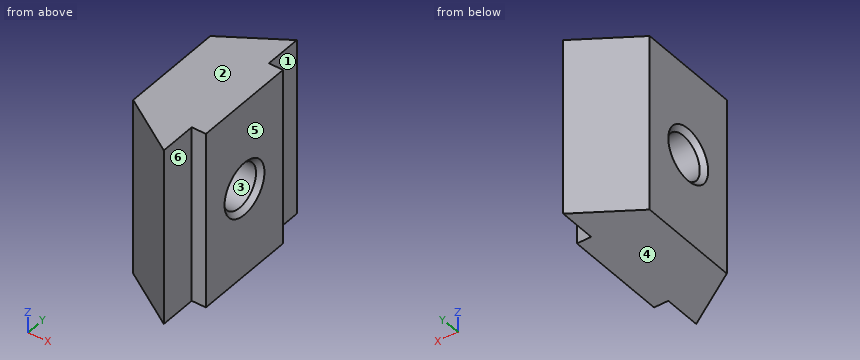
Autodesk Inventor part; units mm, degrees
ref_plane "nut_XY" through (0, 0, 0) normal (1, 0, 0) x (0, 0, -1)
ref_plane "nut_YZ" through (0, 0, 0) normal (0, 0, -1) x (0, 1, 0)
ref_plane "nut_ZX" through (0, 0, 0) normal (0, 1, 0) x (1, 0, 0)
sketch "Sketch_4" plane through (0, 0, 0) normal (0, 0, 1) x (1, 0, 0)
  line L0 (-4.1, 2.9) -> (-4.1, -2.9)
  line L1 (-4.1, -2.9) -> (-0.8, -5)
  line L2 (-0.8, -5) -> (-0.8, -2.9)
  line L3 (-0.8, -2.9) -> (0, -2.9)
  line L4 (0, -2.9) -> (0, 2.9)
  line L5 (0, 2.9) -> (-0.8, 2.9)
  line L6 (-0.8, 2.9) -> (-0.8, 5)
  line L7 (-0.8, 5) -> (-4.1, 2.9)
extrude "Extrusion1" add sketch "Sketch_4" along normal mid plane 10
sketch "Sketch_5" plane through (0, 0, 0) normal (0, 0, 1) x (1, 0, 0)
  line L0 (0, 0) -> (-4.1, 0)
  line L1 (-4.1, 0) -> (-4.1, 1.5)
  line L2 (-4.1, 1.5) -> (-3.8295, 1.2295)
  line L3 (-3.8295, 1.2295) -> (-0.2705, 1.2295)
  line L4 (-0.2705, 1.2295) -> (0, 1.5)
  line L5 (0, 1.5) -> (0, 0)
  line L6 (0, 0) -> (-4.1, 0)
revolve "Revolution1" cut sketch "Sketch_5" angle 360 about axis through (0, 0, 0) along (1, 0, 0)
thread "Thread1"
ref_plane "nut_XY" through (0, 0, 0) normal (1, 0, 0) x (0, 0, -1)
ref_plane "nut_YZ" through (0, 0, 0) normal (0, 0, -1) x (0, 1, 0)
ref_plane "nut_ZX" through (0, 0, 0) normal (0, 1, 0) x (1, 0, 0)
ref_plane "to_bolt_XY" through (-4.1, 0, 0) normal (1, 0, 0) x (0, 0, -1)
ref_plane "to_bolt_YZ" through (-4.1, 0, 0) normal (0, 0, -1) x (0, 1, 0)
ref_plane "to_bolt_ZX" through (-4.1, 0, 0) normal (0, 1, 0) x (1, 0, 0)
ref_plane "to_frames_XY" through (-0.8, 0, 0) normal (1, 0, 0) x (0, 0, -1)
ref_plane "to_frames_YZ" through (-0.8, 0, 0) normal (0, 0, -1) x (0, 1, 0)
ref_plane "to_frames_ZX" through (-0.8, 0, 0) normal (0, 1, 0) x (1, 0, 0)
properties part number "HNTT5-3_1"
Input: part model. Units: mm. Frame: model coordinates. Face numbers are marked on the shaded views. A direction names the side the tool comes from. Coordinates: 2 decimals unless noted, no trailing zeros. Order: outer loops, then holes, each group sorted by start corner. A loop starts at its lowest first (then second) coordinate and runs counter-clockwise, first axis right, second up.
1. Cut plane A-A, the plane y = 0. Return loops of the section in (x, z).
Checked values:
outline: (-4.1, -5) - (0, -5) - (0, -1.5) - (-0.27, -1.23) - (-3.83, -1.23) - (-4.1, -1.5) - close; (-4.1, 1.5) - (-3.83, 1.23) - (-0.27, 1.23) - (0, 1.5) - (0, 5) - (-4.1, 5) - close
2. Cut plane B-B, the plane z = 0. Return loops of the section in (x, y).
Checked values:
outline: (-4.1, -2.9) - (-0.8, -5) - (-0.8, -2.9) - (0, -2.9) - (0, -1.5) - (-0.27, -1.23) - (-3.83, -1.23) - (-4.1, -1.5) - close; (-4.1, 1.5) - (-3.83, 1.23) - (-0.27, 1.23) - (0, 1.5) - (0, 2.9) - (-0.8, 2.9) - (-0.8, 5) - (-4.1, 2.9) - close
3. Ray query, line 1 along Z through (x, y) = (-1.25, 0); line 2 along Y through (x, z) = (-0.5, -2.5); line 3 along Z through (x, y) = (-1.55, -0.5). Return the intervals inside material, ascending.
Checked values:
line 1: z = -5 to -1.23, 1.23 to 5
line 2: y = -2.9 to 2.9
line 3: z = -5 to -1.12, 1.12 to 5
4. Cut plane C-C, the plane x = -3.35. Return loops of the section in (y, z), plus the area to 3 significant figures.
Checked values:
outline: (-3.38, -5) - (3.38, -5) - (3.38, 5) - (-3.38, 5) - close; hole circle Ø2.46 at (0, 0)
area: 62.8 mm2
5. Access query for the marked faces 5 and 6. Directions: +Z, -Z, +X, -X, +Y, -Y. A direction counts if a zero-diameter tool reaches every point of the face in a straight line with its end or side. Return the directions, or none.
Checked values:
face 5: +Z, -Z, +X, +Y, -Y
face 6: +Z, -Z, +X, -Y
6. Contact query for flat-ended pins moving along their axis: P1, Ø2, axis at x = -3.5, z = 3, coming from the +Y side; P2, Ø0.9, axis at x = -0.5, z = 1.5, coming from the -Y side. Output: stop coordinate, or through.
Checked values:
P1: stops at y = 3.92
P2: stops at y = -5
7. Draft query along Z for the marked faces 1, 2, 3 and 4. Return one class per face: +Z half, -Z half, draft (parallel to the pull), parting line (faces both ways), or undercut.
Checked values:
face 1: draft
face 2: +Z half
face 3: undercut
face 4: -Z half
8. Cut plane D-D, the plane x = -1.95. Return loops of the section in (y, z), plus the area to 3 significant figures.
Checked values:
outline: (-4.27, -5) - (4.27, -5) - (4.27, 5) - (-4.27, 5) - close; hole circle Ø2.46 at (0, 0)
area: 80.6 mm2
